For this review, take the finished solid that the model builds, in its own axes (mm). Face numbers are marked on the shaded views. A direction names the side the tool comes from. Coordinates: 2 decimals unless noted, no trailing zeros. Write each loop counter-clockwise with the first axis right and the second up, starting at its lowest first coordinate (ties: lowest second). Pieces come first, ordered by that corner, then holes. Notation, with made-up numbers: M 37,78 L 82,78 A25 ccw 82,116 Z; hole C -21.75,12.25 d7. An arc over 180 degrees is marked long. Return JSON: item names as keys, results as strings.
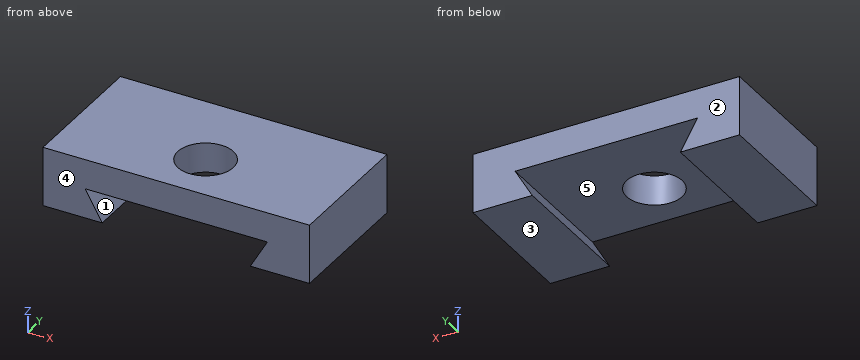
```python
from build123d import *

# Parameters (mm, degrees)
F0_W     = 114.3
F0_H     = 58.7375
F1_DEPTH = 25.4
F3_DEPTH = 70.358
F4_R     = 11.90625
F5_DEPTH = 24.892


with BuildPart() as f1:
    # F0 (on Top) → F1 (new body)
    with BuildSketch(Plane.XY):
        with Locations((-4.318278, 5.723361)):
            Rectangle(F0_W, F0_H)
    extrude(amount=-F1_DEPTH)

    # F2 (on face) → F3 (cut)
    with BuildSketch(Plane.XZ.offset(23.645389)):
        Polygon((-43.400627, -12.7), (-36.068278, -25.4), (27.431722, -25.4), (34.76407, -12.7), align=None)
    extrude(amount=-F3_DEPTH, mode=Mode.SUBTRACT)

    # F4 (on face) → F5 (cut)
    with BuildSketch(Plane.XY):
        with Locations((-4.318278, -1.420389)):
            Circle(F4_R)
    extrude(amount=-F5_DEPTH, mode=Mode.SUBTRACT)


solid = f1.part
```
1. We need section A-A (x = -41). State the section outline as (y, z) points, plus the area to 3 significant figures.
Checks:
{"outline": "M -23.65,-25.4 L 35.09,-25.4 L 35.09,-16.86 L -23.65,-16.86 Z; M -23.65,-12.7 L 35.09,-12.7 L 35.09,0 L -23.65,0 Z", "area": "1,250 mm2"}
2. We need section C-C (z = -17.5). State the section outline as (x, y) points, plus the area to 3 significant figures.
Checks:
{"outline": "M -61.47,-23.65 L -40.63,-23.65 L -40.63,35.09 L -61.47,35.09 Z; M 31.99,-23.65 L 52.83,-23.65 L 52.83,35.09 L 31.99,35.09 Z", "area": "2,450 mm2"}
3. Draft analysis for pull direction Z (two halves, no side actions). For the marked faces 1, 2 and 3, state which applies: +Z half, -Z half, draft (parallel to the pull), parting line (faces both ways), or undercut.
Checks:
{"face 1": "undercut", "face 2": "draft", "face 3": "-Z half"}
4. Wall thickness on L1, parallel to Z at x = -18, y = -3.5; L2, parallel to X at y = 9, z = -4; L3, parallel to X at y = 15.5, z = -22: over which ranges is each line inside the solid? List them lowest first. Write a range as from..to.
Checks:
{"L1": "-12.7..0", "L2": "-61.47..-10.08, 1.44..52.83", "L3": "-61.47..-38.03, 29.39..52.83"}
5. For the marked faces 4 and 5, list the 3-axis set-ups (+Z, -Z, +X, -X, +Y, -Y) from which the entire face can be reached by the end or side of a thin tool; tool diameter is ignored.
Checks:
{"face 4": "+Z, -Z, +X, -X, -Y", "face 5": "+Y, -Y"}
6. Clearance check with a flat-ended pin moving along its axis: pin 1 Ø1.5 at (x, y) = (25, -13) entering from -Z. State where the tip first meets the part, or that it passes through.
Checks:
{"pin 1": "z = -12.7"}
7. We need section B-B (y = -4). State the section outline as (x, z) points.
Checks:
{"outline": "M -61.47,-25.4 L -36.07,-25.4 L -43.4,-12.7 L -15.94,-12.7 L -15.94,0 L -61.47,0 Z; M 7.31,-12.7 L 34.76,-12.7 L 27.43,-25.4 L 52.83,-25.4 L 52.83,0 L 7.31,0 Z"}
8. We need section D-D (y = 15). State the section outline as (x, z) points.
Checks:
{"outline": "M -61.47,-25.4 L -36.07,-25.4 L -43.4,-12.7 L 34.76,-12.7 L 27.43,-25.4 L 52.83,-25.4 L 52.83,0 L -61.47,0 Z"}
